Source: CAD feature listing. Evaluate the final solid. Frame: model axes, mm. Face numbers are marked on the shaded views. Round coordinates to 2 decimals unless told otherwise and drop trailing zeros. Order: outer loops, then holes, each group sorted by start corner. A loop starts at its lowest first (then second) coordinate and runs counter-clockwise, first axis right, second up. Notation, with made-up numbers: M 68,59.5 L 102,59.5 A19 cw 102,63.5 Z; hole C -1,25 d6. An arc over 180 degrees is marked long. Use CSV: the item, a comma, the result in double quotes. Start each with the question number.
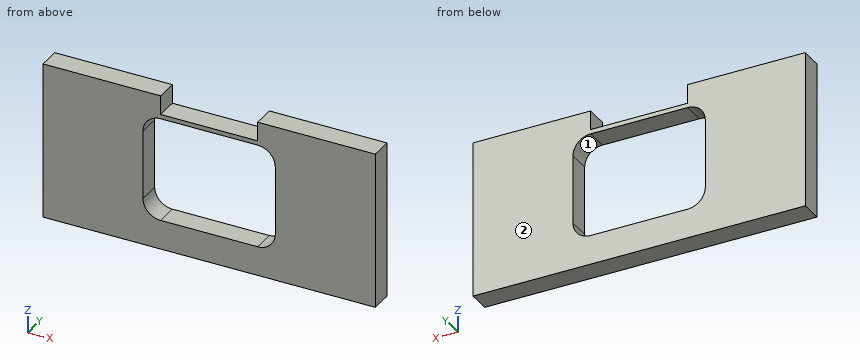
```python
from build123d import *

# Parameters (mm, degrees)
F0_W     = 226
F0_H     = 111
F0_W_2   = 90
F0_H_2   = 71
F1_DEPTH = 15
F2_R     = 12
F4_DEPTH = 25


with BuildPart() as f1:
    # F0 (on Front) → F1 (new body)
    with BuildSketch(Plane.XZ):
        Rectangle(F0_W, F0_H)
        Rectangle(F0_W_2, F0_H_2, mode=Mode.SUBTRACT)
    extrude(amount=F1_DEPTH)

    # F2
    f2_edges = [f1.edges().sort_by_distance(p)[0] for p in [
        (45, -7.5, 35.5),
        (45, -7.5, -35.5),
        (-45, -7.5, -35.5),
        (-45, -7.5, 35.5),
    ]]
    fillet(f2_edges, radius=F2_R)

    # F3 (on face) → F4 (cut)
    with BuildSketch(Plane.XZ.offset(15)):
        Polygon((-33, 51.5), (-33, 47.5), (-33, 38.5), (33, 38.5), (33, 47.5), (33, 51.5), (113, 51.5), (113, 55.5), (-113, 55.5), (-113, 51.5), align=None)
    extrude(amount=-F4_DEPTH, mode=Mode.SUBTRACT)


solid = f1.part
```
(1) Section A-A on x = 22. Return loops of the section in (y, z).
(2) Draft query along X for the marked faces 1 and 2. Return one class per face: pulls with the +X half, pulls with the -X half, needs draft (parallel to the pull), parting line crosses it, or undercut.
(3) Section B-B on y = -6.75. Return loops of the section in (x, z).
(4) Contact query for a flat-ended pin moving along its axis: P1, Ø4.5, axis at x = 7.5, y = -7, coming from the +Z side. Output: stop coordinate, or through.
(5) Line query: line 1 along Z through (x, y) = (11, -10.5); line 2 along X through (y, z) = (-10, -2); line 3 along X through (y, z) = (-11.75, 40.5). Output: solid intervals per line, ascending.
(6) Section C-C on z = 18.5. Return loops of the section in (x, y), plus the area to 3 significant figures.
Results below:
1,outline,"M -15,-55.5 L 0,-55.5 L 0,-35.5 L -15,-35.5 Z; M -15,35.5 L 0,35.5 L 0,38.5 L -15,38.5 Z"
2,face 1,"undercut"
2,face 2,"needs draft"
3,outline,"M -113,-55.5 L 113,-55.5 L 113,51.5 L 33,51.5 L 33,38.5 L -33,38.5 L -33,51.5 L -113,51.5 Z; hole M -45,-23.5 A12 ccw -33,-35.5 L 33,-35.5 A12 ccw 45,-23.5 L 45,23.5 A12 ccw 33,35.5 L -33,35.5 A12 ccw -45,23.5 Z"
4,P1,"stops at z = 38.5"
5,line 1,"z = -55.5 to -35.5, 35.5 to 38.5"
5,line 2,"x = -113 to -45, 45 to 113"
5,line 3,"x = -113 to -33, 33 to 113"
6,outline,"M -113,-15 L -45,-15 L -45,0 L -113,0 Z; M 45,-15 L 113,-15 L 113,0 L 45,0 Z"
6,area,"2,040 mm2"
